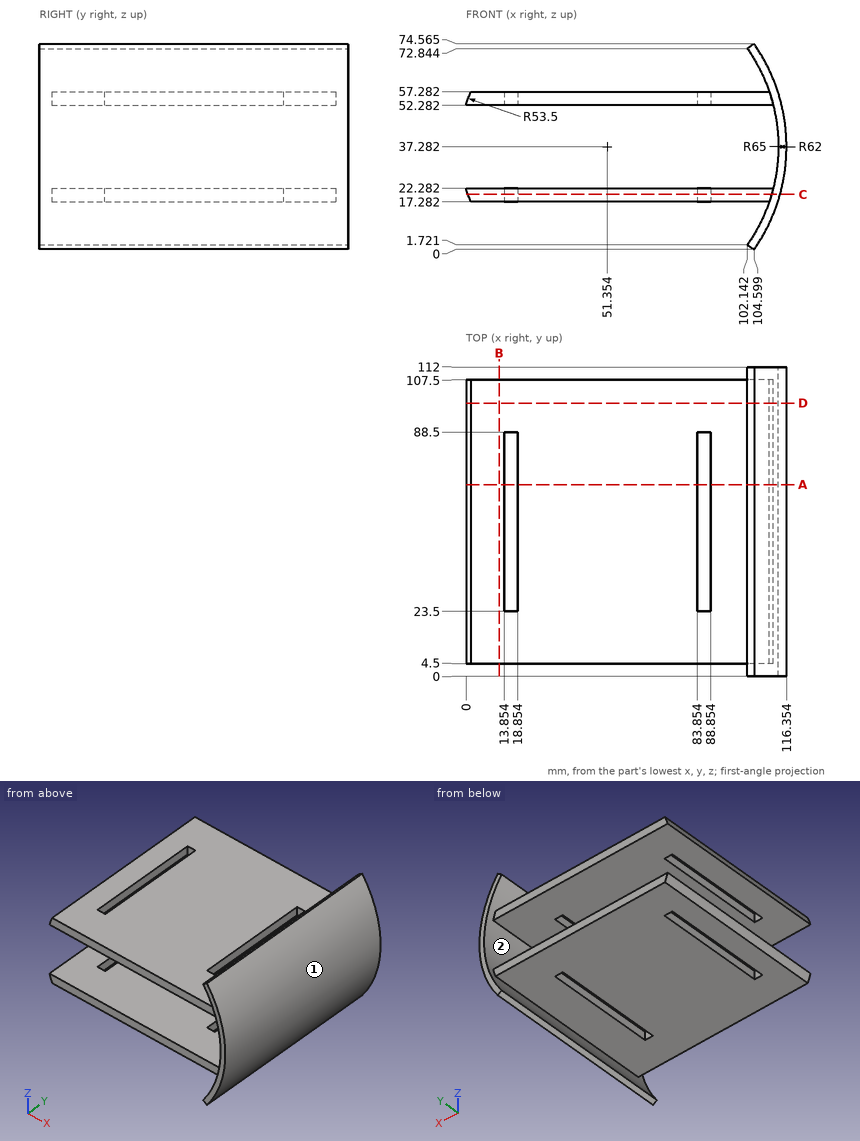
The drawing under review shows one solid part. Ordinate dimensions are in mm from its lowest x, y, z. Give positions to 0.01 mm unless a question says otherwise; leave off trailing zeros. Write each loop counter-clockwise with the first axis right and the second up, starting at its lowest first coordinate (ties: lowest second). Pieces come first, ordered by that corner, then holes. Notation, with made-up numbers: M -26,-40 L -18,-40 A11 cw -18,-19 Z; hole C 38,32.25 d2. An arc over 180 degrees is marked long. Write each question's results on one line, items separated by ' | '. Start each with the question number.
1. Mouldability with a two-part tool opening along Z and no side actions: class the marked faces 1 and 2 as released by +Z, released by -Z, zero draft, split by the parting line, or undercut.
2. We need section B-B (x = 12). Write out the cut boundary in (y, z), and give its area (3 significant figures).
3. We need section C-C (z = 20). Write out the cut boundary in (x, y) (1 decimal), and give its area (3 significant figures).
4. We need section D-D (y = 99). Write out the cut boundary in (x, z) (1 decimal), and give its area (3 significant figures).
5. For probe 1 along Z at (x, y) = (11.5, 32); probe 2 along X at (y, z) = (54, 53.5) (1 decimal); probe 3 along X at (y, z) = (34, 19) (1 decimal), list the stretches that pass through material, from the lowest coordinate up. Write a range as [from, to].
6. Insertion check: pin 1 Ø1.5 at (y, z) = (47.5, 20.5) entering from -X; pin 2 Ø4 at (x, z) = (30.5, 53.5) entering from -Y; pin 3 Ø1.5 at (y, z) = (58, 20.5) entering from +X; pin 4 Ø8 at (x, z) = (27.5, 10) entering from -Y. Each pin has a flat end and moves straight along its axis. Give the tip position at first contact, or say it passes through.
7. We need section A-A (y = 69.5). Write out the cut boundary in (x, z) (1 decimal).
Results found:
1) face 1: split by the parting line | face 2: undercut
2) outline: M 4.5,17.28 L 107.5,17.28 L 107.5,22.28 L 4.5,22.28 Z; M 4.5,52.28 L 107.5,52.28 L 107.5,57.28 L 4.5,57.28 Z | area: 1,030 mm^2
3) outline: M 0.7,4.5 L 110.9,4.5 L 110.9,0 L 114,0 L 114,112 L 110.9,112 L 110.9,107.5 L 0.7,107.5 Z; hole M 13.9,23.5 L 18.9,23.5 L 18.9,88.5 L 13.9,88.5 Z; hole M 83.9,23.5 L 88.9,23.5 L 88.9,88.5 L 83.9,88.5 Z | area: 11,000 mm^2
4) outline: M 0,22.3 A53.5 ccw 1.7,17.3 L 110,17.3 A62 cw 102.1,1.7 L 104.6,0 A65 ccw 104.6,74.6 L 102.1,72.8 A62 cw 110,57.3 L 1.7,57.3 A53.5 ccw 0,52.3 L 111.5,52.3 A62 cw 111.5,22.3 Z | area: 1,330 mm^2
5) probe 1: z = [17.28, 22.28], [52.28, 57.28] | probe 2: x = [0.4, 13.9], [18.9, 83.9], [88.9, 114.3] | probe 3: x = [1.1, 13.9], [18.9, 83.9], [88.9, 113.7]
6) pin 1: stops at x = 0.31 | pin 2: stops at y = 4.5 | pin 3: stops at x = 114.35 | pin 4: passes through
7) outline: M 0,22.3 A53.5 ccw 1.7,17.3 L 13.9,17.3 L 13.9,22.3 Z; M 0,52.3 L 13.9,52.3 L 13.9,57.3 L 1.7,57.3 A53.5 ccw Z; M 18.9,17.3 L 83.9,17.3 L 83.9,22.3 L 18.9,22.3 Z; M 18.9,52.3 L 83.9,52.3 L 83.9,57.3 L 18.9,57.3 Z; M 88.9,17.3 L 110,17.3 A62 cw 102.1,1.7 L 104.6,0 A65 ccw 104.6,74.6 L 102.1,72.8 A62 cw 110,57.3 L 88.9,57.3 L 88.9,52.3 L 111.5,52.3 A62 cw 111.5,22.3 L 88.9,22.3 Z
